Could you check a few things on this model? Use its own coordinates, in mm. Face numbers are marked on the shaded views. A direction names the side the tool comes from. Coordinates: 2 decimals unless noted, no trailing zeros. Order: outer loops, then holes, each group sorted by start corner. A loop starts at its lowest first (then second) coordinate and runs counter-clockwise, first axis right, second up. Notation, with made-up numbers: (30, 52) -> (43, 52) arc R22 ccw to (43, 75) -> close; hole circle Ø7 at (83.5, 13.25). An arc over 180 degrees is marked (long way). Put each result on its own line as item: value. Start each with the question number.
Q1. If we section it at A-A (z = 0): Please give me the cut outline in (x, y).
Q2. Will these pins go through, and if not, where does the flat tip stop? pin 1 (3.5 mm diameter, centred on x = 25, z = 5, fed in from +Y); pin 2 (7.5 mm diameter, centred on x = 4, z = -5, fed in from +Y); pin 3 (2 mm diameter, centred on y = 5, z = -12.5, fed in from +X); pin 4 (2 mm diameter, centred on y = 1.5, z = -25.5, fed in from -X).
Q3. We'd pull the mould along Z, two halves only. Please class the marked faces 1, 2 and 3: +Z half, -Z half, draft (parallel to the pull), parting line (faces both ways), or undercut.
Q4. If we section it at B-B (y = 1): Count the separate pieces of the cut face and the enclosed holes in it, and give its area (3 significant figures).
Q5. For the marked faces 4, 5 and 6, which set-ups out of +Z, -Z, +X, -X, +Y, -Y let a thin tool reach every point of the face, with its end or its side?
Q6. If we section it at D-D (z = -25): Please give me the cut outline in (x, y).
Q7. Please list where these lines run through material, in increasing order: line 1 along X through (y, z) = (1.7, 0); line 2 along Z through (x, y) = (-6, 7.75); line 3 along Y through (x, z) = (12.5, -22.5).
Q8. If we section it at C-C (x = 0): Please give me the cut outline in (y, z), and give its area (3 significant figures).
from build123d import *

# Parameters (mm, degrees)
SKETCH_1_R               = 11.5
SKETCH_1_R_2             = 1.5
EXTRUDE_1_DEPTH          = 2.5
SKETCH_2_R               = 12.5
EXTRUDE_2_DEPTH          = 6
HOLE_WIZARD_M3_1_REACH   = 61.651
HOLE_WIZARD_M3_1_BORE_R  = 1.25
PATTERN_CIRCULAR_1_COUNT = 4


with BuildPart() as part:
    # 草图1 → 凸台-拉伸1 (new body)
    with BuildSketch(Plane(origin=(0, 0, 0), x_dir=(1, 0, 0), z_dir=(0, 1, 0))):
        with BuildLine():
            Line((-11.5, 29.5), (11.5, 29.5))
            ThreePointArc((11.5, 29.5), (12.914213562, 28.914213562), (13.5, 27.5))
            Line((13.5, 27.5), (13.5, 21.5))
            ThreePointArc((13.5, 21.5), (15.843145751, 15.843145751), (21.5, 13.5))
            Line((21.5, 13.5), (27.5, 13.5))
            ThreePointArc((27.5, 13.5), (28.914213562, 12.914213562), (29.5, 11.5))
            Line((29.5, 11.5), (29.5, -11.5))
            ThreePointArc((29.5, -11.5), (28.914213562, -12.914213562), (27.5, -13.5))
            Line((27.5, -13.5), (21.5, -13.5))
            ThreePointArc((21.5, -13.5), (15.843145751, -15.843145751), (13.5, -21.5))
            Line((13.5, -21.5), (13.5, -27.5))
            ThreePointArc((13.5, -27.5), (12.914213562, -28.914213562), (11.5, -29.5))
            Line((11.5, -29.5), (-11.5, -29.5))
            ThreePointArc((-11.5, -29.5), (-12.914213562, -28.914213562), (-13.5, -27.5))
            Line((-13.5, -27.5), (-13.5, -21.5))
            ThreePointArc((-13.5, -21.5), (-15.843145751, -15.843145751), (-21.5, -13.5))
            Line((-21.5, -13.5), (-27.5, -13.5))
            ThreePointArc((-27.5, -13.5), (-28.914213562, -12.914213562), (-29.5, -11.5))
            Line((-29.5, -11.5), (-29.5, 11.5))
            ThreePointArc((-29.5, 11.5), (-28.914213562, 12.914213562), (-27.5, 13.5))
            Line((-27.5, 13.5), (-21.5, 13.5))
            ThreePointArc((-21.5, 13.5), (-15.843145751, 15.843145751), (-13.5, 21.5))
            Line((-13.5, 21.5), (-13.5, 27.5))
            ThreePointArc((-13.5, 27.5), (-12.914213562, 28.914213562), (-11.5, 29.5))
        make_face()
        with Locations(Location((0, 0, 0), (0, 0, 270))):
            Circle(SKETCH_1_R, mode=Mode.SUBTRACT)
        with Locations(Location((-5, 25, 0), (0, 0, 270))):
            Circle(SKETCH_1_R_2, mode=Mode.SUBTRACT)
        with Locations(Location((5, 25, 0), (0, 0, 90))):
            Circle(SKETCH_1_R_2, mode=Mode.SUBTRACT)
        with Locations(Location((25, 5, 0), (0, 0, 270))):
            Circle(SKETCH_1_R_2, mode=Mode.SUBTRACT)
        with Locations(Location((25, -5, 0), (0, 0, 90))):
            Circle(SKETCH_1_R_2, mode=Mode.SUBTRACT)
        with Locations(Location((5, -25, 0), (0, 0, 270))):
            Circle(SKETCH_1_R_2, mode=Mode.SUBTRACT)
        with Locations(Location((-5, -25, 0), (0, 0, 90))):
            Circle(SKETCH_1_R_2, mode=Mode.SUBTRACT)
        with Locations(Location((-25, -5, 0), (0, 0, 270))):
            Circle(SKETCH_1_R_2, mode=Mode.SUBTRACT)
        with Locations(Location((-25, 5, 0), (0, 0, 90))):
            Circle(SKETCH_1_R_2, mode=Mode.SUBTRACT)
    extrude(amount=EXTRUDE_1_DEPTH)

    # 草图2 → 凸台-拉伸2 (add)
    with BuildSketch(Plane(origin=(0, 2.5, 0), x_dir=(1, 0, 0), z_dir=(0, 1, 0))):
        Polygon((17.5, 7.5), (7.5, 17.5), (-7.5, 17.5), (-17.5, 7.5), (-17.5, -7.5), (-7.5, -17.5), (7.5, -17.5), (17.5, -7.5), align=None)
        with Locations(Location((0, 0, 0), (0, 0, 270))):
            Circle(SKETCH_2_R, mode=Mode.SUBTRACT)
    extrude(amount=EXTRUDE_2_DEPTH)

    # M3 螺纹孔1 bore (on position points) → M3 螺纹孔1 (cut, up to next)
    with BuildSketch(Plane(origin=(-12.5, 5.5, 12.5), x_dir=(0.707106781187, 0, 0.707106781187), z_dir=(-0.707106781187, 0, 0.707106781187)), mode=Mode.PRIVATE) as hole_wizard_m3_1_sk1:
        Circle(HOLE_WIZARD_M3_1_BORE_R)
    hole_wizard_m3_1_tool1 = extrude(hole_wizard_m3_1_sk1.sketch, amount=-HOLE_WIZARD_M3_1_REACH, mode=Mode.PRIVATE) & part.part
    hole_wizard_m3_1 = hole_wizard_m3_1_tool1.solids().sort_by_distance((-12.5, 5.5, 12.5))[0]
    add(hole_wizard_m3_1, mode=Mode.SUBTRACT)

    # 阵列(圆周)1: M3 螺纹孔1 ×4 about axis
    pattern_circular_1_axis = Axis((0, 8.5, 0), (0, -1, 0))
    for i in range(1, PATTERN_CIRCULAR_1_COUNT):
        add(hole_wizard_m3_1.rotate(pattern_circular_1_axis, i * 360 / PATTERN_CIRCULAR_1_COUNT), mode=Mode.SUBTRACT)


solid = part.part
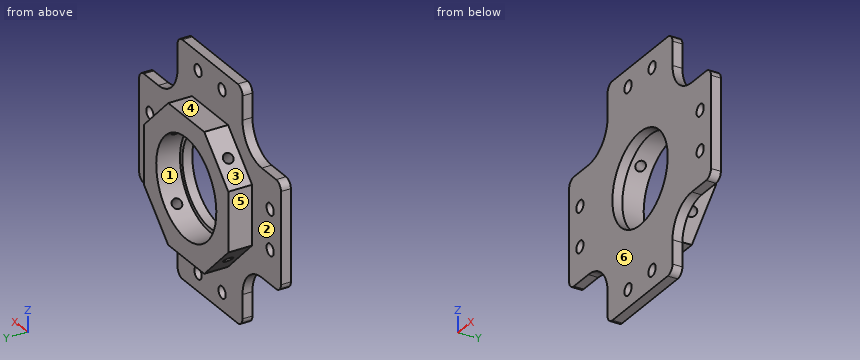
The answers:
1. outline: (-29.5, 0) -> (-11.5, 0) -> (-11.5, 2.5) -> (-12.5, 2.5) -> (-12.5, 8.5) -> (-17.5, 8.5) -> (-17.5, 2.5) -> (-29.5, 2.5) -> close; (11.5, 0) -> (29.5, 0) -> (29.5, 2.5) -> (17.5, 2.5) -> (17.5, 8.5) -> (12.5, 8.5) -> (12.5, 2.5) -> (11.5, 2.5) -> close
2. pin 1: y = 2.5
2. pin 2: through
2. pin 3: x = 13.5
2. pin 4: x = -13.5
3. face 1: undercut
3. face 2: draft
3. face 3: +Z half
4. separate pieces: 1
4. enclosed holes: 9
4. area: 2,030 mm^2
5. face 4: +Z, +X, -X, +Y
5. face 5: +Z, -Z, -X, +Y
5. face 6: +Z, -Z, +X, -X, -Y
6. outline: (-13.5, 0) -> (-6.5, 0) -> (-6.5, 2.5) -> (-13.5, 2.5) -> close; (-3.5, 0) -> (3.5, 0) -> (3.5, 2.5) -> (-3.5, 2.5) -> close; (6.5, 0) -> (13.5, 0) -> (13.5, 2.5) -> (6.5, 2.5) -> close
7. line 1: -29.5 to -11.5, 11.5 to 29.5
7. line 2: -17.5 to -10.97, 10.97 to 17.5
7. line 3: 0 to 2.5
8. outline: (0, -29.5) -> (2.5, -29.5) -> (2.5, -17.5) -> (8.5, -17.5) -> (8.5, -12.5) -> (2.5, -12.5) -> (2.5, -11.5) -> (0, -11.5) -> close; (0, 11.5) -> (2.5, 11.5) -> (2.5, 12.5) -> (8.5, 12.5) -> (8.5, 17.5) -> (2.5, 17.5) -> (2.5, 29.5) -> (0, 29.5) -> close
8. area: 150 mm^2
